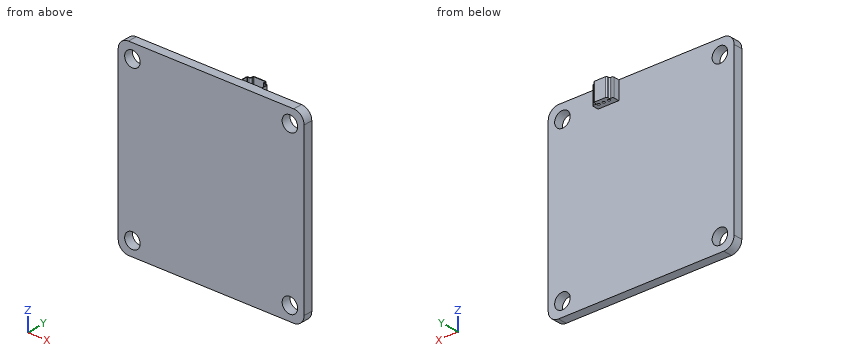
```python
from build123d import *

# Parameters (mm, degrees)
SKETCH1_R           = 1.5
BOSS_EXTRUDE1_DEPTH = 1.75
BOSS_EXTRUDE2_DEPTH = 3
BOSS_EXTRUDE3_DEPTH = 0.5
CUT_EXTRUDE1_REACH  = 5.5
SKETCH4_R           = 0.25


with BuildPart() as part:
    # Sketch1 → Boss-Extrude1 (new body)
    with BuildSketch(Plane(origin=(0, 0, 0), x_dir=(1, 0, 0), z_dir=(0, 1, 0))):
        with BuildLine():
            Line((16, -18), (-16, -18))
            ThreePointArc((-16, -18), (-17.414213562, -17.414213562), (-18, -16))
            Line((-18, -16), (-18, 16))
            ThreePointArc((-18, 16), (-17.414213562, 17.414213562), (-16, 18))
            Line((-16, 18), (16, 18))
            ThreePointArc((16, 18), (17.414213562, 17.414213562), (18, 16))
            Line((18, 16), (18, -16))
            ThreePointArc((18, -16), (17.414213562, -17.414213562), (16, -18))
        make_face()
        with Locations((-15.25, 15.25)):
            Circle(SKETCH1_R, mode=Mode.SUBTRACT)
        with Locations((15.25, 15.25)):
            Circle(SKETCH1_R, mode=Mode.SUBTRACT)
        with Locations((15.25, -15.25)):
            Circle(SKETCH1_R, mode=Mode.SUBTRACT)
        with Locations((-15.25, -15.25)):
            Circle(SKETCH1_R, mode=Mode.SUBTRACT)
    extrude(amount=BOSS_EXTRUDE1_DEPTH)

    # Sketch2 → Boss-Extrude2 (add)
    with BuildSketch(Plane.XY.offset(18)):
        with BuildLine():
            Line((4.325932744, 1.75), (8.325932744, 1.75))
            Line((8.325932744, 1.75), (8.325932744, 2.893191045))
            ThreePointArc((8.325932744, 2.893191045), (8.2673541, 3.034612401), (8.125932744, 3.093191045))
            Line((8.125932744, 3.093191045), (7.710555572, 3.093191045))
            ThreePointArc((7.710555572, 3.093191045), (7.569134216, 3.151769689), (7.510555572, 3.293191045))
            Line((7.510555572, 3.293191045), (7.510555572, 3.55))
            ThreePointArc((7.510555572, 3.55), (7.451976928, 3.691421356), (7.310555572, 3.75))
            Line((7.310555572, 3.75), (5.170220599, 3.75))
            ThreePointArc((5.170220599, 3.75), (5.028799243, 3.691421356), (4.970220599, 3.55))
            Line((4.970220599, 3.55), (4.970220599, 3.293191045))
            ThreePointArc((4.970220599, 3.293191045), (4.911641955, 3.151769689), (4.770220599, 3.093191045))
            Line((4.770220599, 3.093191045), (4.525932744, 3.093191045))
            ThreePointArc((4.525932744, 3.093191045), (4.384511387, 3.034612401), (4.325932744, 2.893191045))
            Line((4.325932744, 2.893191045), (4.325932744, 1.75))
        make_face()
        with BuildLine():
            Line((4.425932744, 1.85), (8.225932744, 1.85))
            Line((8.225932744, 1.85), (8.225932744, 2.893191045))
            ThreePointArc((8.225932744, 2.893191045), (8.196643422, 2.963901723), (8.125932744, 2.993191045))
            Line((8.125932744, 2.993191045), (7.710555572, 2.993191045))
            ThreePointArc((7.710555572, 2.993191045), (7.498423538, 3.081059011), (7.410555572, 3.293191045))
            Line((7.410555572, 3.293191045), (7.410555572, 3.55))
            ThreePointArc((7.410555572, 3.55), (7.38126625, 3.620710678), (7.310555572, 3.65))
            Line((7.310555572, 3.65), (5.170220599, 3.65))
            ThreePointArc((5.170220599, 3.65), (5.099509921, 3.620710678), (5.070220599, 3.55))
            Line((5.070220599, 3.55), (5.070220599, 3.293191045))
            ThreePointArc((5.070220599, 3.293191045), (4.982352633, 3.081059011), (4.770220599, 2.993191045))
            Line((4.770220599, 2.993191045), (4.525932744, 2.993191045))
            ThreePointArc((4.525932744, 2.993191045), (4.455222065, 2.963901723), (4.425932744, 2.893191045))
            Line((4.425932744, 2.893191045), (4.425932744, 1.85))
        make_face(mode=Mode.SUBTRACT)
    extrude(amount=-BOSS_EXTRUDE2_DEPTH)

    # Sketch3 → Boss-Extrude3 (add)
    with BuildSketch(Plane(origin=(0, 0, 15), x_dir=(-1, 0, 0), z_dir=(0, 0, -1))):
        with BuildLine():
            Line((-4.325932744, 1.75), (-4.325932744, 2.893191045))
            ThreePointArc((-4.325932744, 2.893191045), (-4.384511387, 3.034612401), (-4.525932744, 3.093191045))
            Line((-4.525932744, 3.093191045), (-4.770220599, 3.093191045))
            ThreePointArc((-4.770220599, 3.093191045), (-4.911641955, 3.151769689), (-4.970220599, 3.293191045))
            Line((-4.970220599, 3.293191045), (-4.970220599, 3.55))
            ThreePointArc((-4.970220599, 3.55), (-5.028799243, 3.691421356), (-5.170220599, 3.75))
            Line((-5.170220599, 3.75), (-7.310555572, 3.75))
            ThreePointArc((-7.310555572, 3.75), (-7.451976928, 3.691421356), (-7.510555572, 3.55))
            Line((-7.510555572, 3.55), (-7.510555572, 3.293191045))
            ThreePointArc((-7.510555572, 3.293191045), (-7.569134216, 3.151769689), (-7.710555572, 3.093191045))
            Line((-7.710555572, 3.093191045), (-8.125932744, 3.093191045))
            ThreePointArc((-8.125932744, 3.093191045), (-8.2673541, 3.034612401), (-8.325932744, 2.893191045))
            Line((-8.325932744, 2.893191045), (-8.325932744, 1.75))
            Line((-8.325932744, 1.75), (-4.325932744, 1.75))
        make_face()
    extrude(amount=BOSS_EXTRUDE3_DEPTH)

    # Sketch4 → Cut-Extrude1 (cut, up to next)
    with BuildSketch(Plane(origin=(0, 0, 14.5), x_dir=(-1, 0, 0), z_dir=(0, 0, -1)), mode=Mode.PRIVATE) as cut_extrude1_sk1:
        with Locations((-7.325932744, 2.817782328)):
            Circle(SKETCH4_R)
    cut_extrude1_tool1 = extrude(cut_extrude1_sk1.sketch, amount=-CUT_EXTRUDE1_REACH, mode=Mode.PRIVATE) & part.part
    add(cut_extrude1_tool1.solids().sort_by_distance((7.325933, 2.817782, 14.5))[0], mode=Mode.SUBTRACT)
    # Sketch4 → Cut-Extrude1 (cut, up to next)
    with BuildSketch(Plane(origin=(0, 0, 14.5), x_dir=(-1, 0, 0), z_dir=(0, 0, -1)), mode=Mode.PRIVATE) as cut_extrude1_sk2:
        with Locations((-6.325932744, 2.817782328)):
            Circle(SKETCH4_R)
    cut_extrude1_tool2 = extrude(cut_extrude1_sk2.sketch, amount=-CUT_EXTRUDE1_REACH, mode=Mode.PRIVATE) & part.part
    add(cut_extrude1_tool2.solids().sort_by_distance((6.325933, 2.817782, 14.5))[0], mode=Mode.SUBTRACT)
    # Sketch4 → Cut-Extrude1 (cut, up to next)
    with BuildSketch(Plane(origin=(0, 0, 14.5), x_dir=(-1, 0, 0), z_dir=(0, 0, -1)), mode=Mode.PRIVATE) as cut_extrude1_sk3:
        with Locations((-5.325932744, 2.817782328)):
            Circle(SKETCH4_R)
    cut_extrude1_tool3 = extrude(cut_extrude1_sk3.sketch, amount=-CUT_EXTRUDE1_REACH, mode=Mode.PRIVATE) & part.part
    add(cut_extrude1_tool3.solids().sort_by_distance((5.325933, 2.817782, 14.5))[0], mode=Mode.SUBTRACT)


solid = part.part
```
The listing builds one solid part. Answer for the finished solid, in the listing's coordinates (mm). Give positions to 0.01 mm unless a question says otherwise; leave off trailing zeros. Write each loop counter-clockwise with the first axis right and the second up, starting at its lowest first coordinate (ties: lowest second). Pieces come first, ordered by that corner, then holes. Notation, with made-up numbers: (-18, 40) -> (36, 40) arc R18 ccw to (36, 63) -> close; hole circle Ø3 at (-40, -6). An arc over 180 degrees is marked (long way). Write item = value, one per line. Start each with the question number.
1) Straight lines are drawn through the part: line 1 along Z through (x, y) = (15.25, 1.25); line 2 along Y through (x, z) = (-12.5, -4.5). For each, find the intervals that lie inside material, in ascending order.
2) The part is cut by section A-A, the plane y = 0.55. Determine the outline of the cut face in (x, z), and give its area (3 significant figures).
3) The part is cut by section D-D, the plane z = -6. Determine the outline of the cut face in (x, y).
4) The part is cut by section C-C, the plane z = -15.25. Determine the outline of the cut face in (x, y), and give its area (3 significant figures).
5) The part is cut by section B-B, the plane x = 15.25. Determine the outline of the cut face in (y, z).
6) Each of these flat-tipped pins is pushed along its axis until it touches: pin 1 (12 mm diameter, centred on x = -8, z = 8, fed in from +Y); pin 2 (0.9 mm diameter, centred on y = 2.5, z = 15.5, fed in from +X); pin 3 (1 mm diameter, centred on x = -10.5, z = -1, fed in from -Y); pin 4 (0.9 mm diameter, centred on x = 6.5, y = 2.5, fed in from +Z). Where does it stop, or does it pass through?
Solutions:
q1.line_1 = -18 to -16.75, -13.75 to 13.75, 16.75 to 18
q1.line_2 = 0 to 1.75
q2.outline = (-18, -16) arc R2 ccw to (-16, -18) -> (16, -18) arc R2 ccw to (18, -16) -> (18, 16) arc R2 ccw to (16, 18) -> (-16, 18) arc R2 ccw to (-18, 16) -> close; hole circle Ø3 at (-15.25, -15.25); hole circle Ø3 at (-15.25, 15.25); hole circle Ø3 at (15.25, -15.25); hole circle Ø3 at (15.25, 15.25)
q2.area = 1,260 mm²
q3.outline = (-18, 0) -> (18, 0) -> (18, 1.75) -> (-18, 1.75) -> close
q4.outline = (-18, 0) -> (-16.75, 0) -> (-16.75, 1.75) -> (-18, 1.75) -> close; (-13.75, 0) -> (13.75, 0) -> (13.75, 1.75) -> (-13.75, 1.75) -> close; (16.75, 0) -> (18, 0) -> (18, 1.75) -> (16.75, 1.75) -> close
q4.area = 52.5 mm²
q5.outline = (0, -18) -> (1.75, -18) -> (1.75, -16.75) -> (0, -16.75) -> close; (0, -13.75) -> (1.75, -13.75) -> (1.75, 13.75) -> (0, 13.75) -> close; (0, 16.75) -> (1.75, 16.75) -> (1.75, 18) -> (0, 18) -> close
q6.pin_1 = 1.75
q6.pin_2 = 8.33
q6.pin_3 = 0
q6.pin_4 = 15
